```python
from build123d import *

# Parameters (mm, degrees)
CIRPATTERN1_COUNT = 16
CIRPATTERN2_COUNT = 16


with BuildPart() as part:
    # Sketch1 → Revolve1 (revolve)
    with BuildSketch(Plane.XY, mode=Mode.PRIVATE) as revolve1_sk:
        Polygon((0, 162.5), (0, 127), (17, 110), (43, 110), (43, 143.5), (24, 162.5), align=None)
    revolve(revolve1_sk.sketch.rotate(Axis((0, 0, 0), (1, 0, 0)), 90), axis=Axis((0, 0, 0), (1, 0, 0)))

    # Sketch4 → M12 Tapped Hole1 (revolve, cut)
    with BuildSketch(Plane.ZX.offset(152)):
        Polygon((0, 0), (0, 26.314389157), (5.1, 23.25), (5.1, 0.925), (6.025, 0), align=None)
    m12_tapped_hole1 = revolve(axis=Axis((-6.35, 152, 0), (1, 0, 0)), mode=Mode.SUBTRACT)

    # CirPattern1: M12 Tapped Hole1 ×16 about axis
    cirpattern1_axis = Axis((0, 0, 0), (1, 0, 0))
    for i in range(1, CIRPATTERN1_COUNT):
        add(m12_tapped_hole1.rotate(cirpattern1_axis, i * 360 / CIRPATTERN1_COUNT), mode=Mode.SUBTRACT)

    # Sketch6 → M12 Tapped Hole2 (revolve, cut)
    with BuildSketch(Plane(origin=(43, 129.954049653, 25.849467667), x_dir=(0, 0, -1), z_dir=(0, 1, 0))):
        Polygon((0, 0), (0, 32.314389157), (5.1, 29.25), (5.1, 0.925), (6.025, 0), align=None)
    m12_tapped_hole2 = revolve(axis=Axis((49.35, 129.954049653, 25.849467667), (-1, 0, 0)), mode=Mode.SUBTRACT)

    # CirPattern2: M12 Tapped Hole2 ×16 about axis
    cirpattern2_axis = Axis((0, 0, 0), (1, 0, 0))
    for i in range(1, CIRPATTERN2_COUNT):
        add(m12_tapped_hole2.rotate(cirpattern2_axis, i * 360 / CIRPATTERN2_COUNT), mode=Mode.SUBTRACT)


solid = part.part
```
Part model, mm, in its own coordinate system. A direction names the side the tool comes from. Give positions to 0.01 mm unless a question says otherwise; leave off trailing zeros. Use CSV: the item, a comma, the result in double quotes.
Item 1: Pin check, flat tips, straight feed: P1, Ø16.5, axis at y = 58.17, z = 140.43, coming from the +X side; P2, Ø8, axis at y = -140.43, z = 58.17, coming from the -X side; P3, Ø8, axis at x = 38, z = 71.5, coming from the +Y side. Stop position of each tip, or through.
Taken from the geometry:
P1,"stops at x = 42.75"
P2,"stops at x = 23.91"
P3,"stops at y = 135.16"
Item 2: Drill centre lines: probe 1 along Z at (x, y) = (20, 145); probe 2 along Z at (x, y) = (38.5, 24); probe 3 along Z at (x, y) = (23.5, 57). Where is each one in solid material? Low to high.
Taken from the geometry:
probe 1,"z = -73.36 to -60.43, -55.9 to 55.9, 60.43 to 73.36"
probe 2,"z = -146.04 to -134.71, -125.2 to -107.35, 107.35 to 125.2, 134.71 to 146.04"
probe 3,"z = -152.18 to -144.97, -135.89 to -94.08, 94.08 to 135.89, 144.97 to 152.18"
Item 3: Which spindle directions (+Z, -Z, +X, -X, +Y, -Y) get a long thin tool onto all of the face, cutting with end or side? Do faces 1 (the face through (28.111, 23.301, 125.536)), 2 (the face through (11.931, 62.074, -143.709)). Say none if no direction does.
Taken from the geometry:
face 1,"+X"
face 2,"-X"
